Geometry check sheet. Reference: the model listing, model coordinates, mm. Face numbers are marked on the shaded views. A direction names the side the tool comes from. Give positions to 0.01 mm unless a question says otherwise; leave off trailing zeros. Loops run counter-clockwise (first coordinate to the right, second up) from the corner with the lowest first, then second, coordinate; pieces in that order, holes last.
```python
from build123d import *

# Parameters (mm, degrees)
ESQUISSE1_R        = 4
BOSS_EXTRU_1_DEPTH = 6


with BuildPart() as part:
    # Esquisse1 → Boss.-Extru.1 (new body)
    with BuildSketch(Plane.XY):
        with BuildLine():
            Line((-13.404461185, 2.593779068), (1.595538815, 2.593779068))
            Line((1.595538815, 2.593779068), (1.595538815, 8.593779068))
            Line((1.595538815, 8.593779068), (21.595538815, 8.593779068))
            Line((21.595538815, 8.593779068), (21.595538815, 2.593779068))
            Line((21.595538815, 2.593779068), (36.595538815, 2.593779068))
            Line((36.595538815, 2.593779068), (36.595538815, 8.593779068))
            Line((36.595538815, 8.593779068), (46.595538815, 8.593779068))
            Line((46.595538815, 8.593779068), (46.595538815, 12.048496629))
            ThreePointArc((46.595538815, 12.048496629), (46.383875367, 14.095071218), (45.757845305, 16.0550088))
            Line((45.757845305, 16.0550088), (32.398093908, 46.60680341))
            ThreePointArc((32.398093908, 46.60680341), (15.328741232, 58.554348238), (-3.102903491, 48.839354618))
            Line((-3.102903491, 48.839354618), (-21.992653394, 17.171284404))
            ThreePointArc((-21.992653394, 17.171284404), (-23.045050433, 14.705381827), (-23.404461185, 12.048496629))
            Line((-23.404461185, 12.048496629), (-23.404461185, 8.593779068))
            Line((-23.404461185, 8.593779068), (-13.404461185, 8.593779068))
            Line((-13.404461185, 8.593779068), (-13.404461185, 2.593779068))
        make_face()
        with Locations((14.073480927, 38.593779068)):
            Circle(ESQUISSE1_R, mode=Mode.SUBTRACT)
    extrude(amount=BOSS_EXTRU_1_DEPTH)


solid = part.part
```
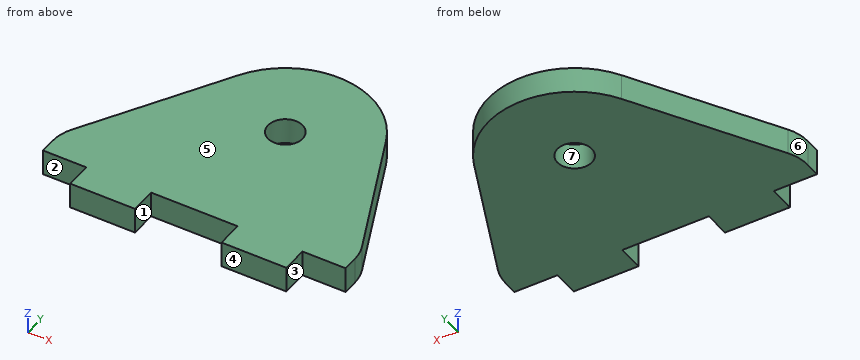
1) Scan lines: line 1 along X through (y, z) = (39, 4); line 2 along X through (y, z) = (38.5, 2.9); line 3 along Y through (x, z) = (34.5, 4.1). Record each from-to range of solid material in increasing order.
2) Sectioned sample at B-B on x = 17. Enter the section's corners in (y, z).
3) Depth check by flat-ended pin: P1, Ø3, axis at y = 5.5, z = 3.5, coming from the -X side; P2, Ø1.5, axis at x = -10.5, z = 1, coming from the +Y side; P3, Ø1.8, axis at x = 40.5, z = 4, coming from the -Y side. Enter the tip coordinate at first touch or a pass-through.
4) Mould release check, pull along Y, two halves, no side actions. Record for the marked faces 4, 5, 6 and 7: +Y half, -Y half, draft (parallel to the pull), parting line (faces both ways), or undercut.
5) Sectioned sample at C-C on z = 2.85. Enter the section's corners in (x, y) (1 decimal).
6) Sectioned sample at A-A on y = 37. Enter the section's corners in (x, z), plus the area to 3 significant figures.
7) Sectioned sample at D-D on x = 41. Enter the section's corners in (y, z), plus the area to 3 significant figures.
8) Tool access check on the marked faces 1, 2 and 3. Record the directions out of +Z, -Z, +X, -X, +Y, -Y that give a thin tool (end or side, any length) a straight path to the whole face; none if there is none.
Determined:
1. line 1: x = -8.97 to 10.09, 18.05 to 35.72
1. line 2: x = -9.27 to 10.07, 18.07 to 35.94
1. line 3: y = 2.59 to 41.8
2. outline: (8.59, 0) - (35.87, 0) - (35.87, 6) - (8.59, 6) - close; (41.32, 0) - (58.38, 0) - (58.38, 6) - (41.32, 6) - close
3. P1: stops at x = -13.4
3. P2: stops at y = 37.7
3. P3: stops at y = 8.59
4. face 4: -Y half
4. face 5: draft
4. face 6: +Y half
4. face 7: undercut
5. outline: (-23.4, 8.6) - (-13.4, 8.6) - (-13.4, 2.6) - (1.6, 2.6) - (1.6, 8.6) - (21.6, 8.6) - (21.6, 2.6) - (36.6, 2.6) - (36.6, 8.6) - (46.6, 8.6) - (46.6, 12) arc R10 ccw to (45.8, 16.1) - (32.4, 46.6) arc R20 ccw to (-3.1, 48.8) - (-22, 17.2) arc R10 ccw to (-23.4, 12) - close; hole circle Ø8 at (14.1, 38.6)
6. outline: (-10.16, 0) - (10.4, 0) - (10.4, 6) - (-10.16, 6) - close; (17.74, 0) - (36.6, 0) - (36.6, 6) - (17.74, 6) - close
6. area: 237 mm2
7. outline: (8.59, 0) - (26.94, 0) - (26.94, 6) - (8.59, 6) - close
7. area: 110 mm2
8. face 1: +Z, -Z, -Y
8. face 2: +Z, -Z, -X, -Y
8. face 3: +Z, -Z, +X, -Y
